Read the model definition and answer for the solid it produces. Units are mm, in the model's axes. Give positions to 0.01 mm unless a question says otherwise; leave off trailing zeros. Order: outer loops, then holes, each group sorted by start corner. A loop starts at its lowest first (then second) coordinate and runs counter-clockwise, first axis right, second up. Notation, with made-up numbers: (54, 26) -> (81, 26) arc R30 cw to (81, 62) -> close; hole circle Ø4 at (-6.5, 74.25). An arc over 180 degrees is marked (long way). One line per item, written item: value. Start each with the question number.
from build123d import *

# Parameters (mm, degrees)
SKETCH2_R           = 11
BOSS_EXTRUDE1_DEPTH = 7.5
SKETCH3_R           = 4.15
SKETCH3_R_2         = 1.25
CUT_EXTRUDE1_DEPTH  = 8.5


with BuildPart() as part:
    # Sketch2 → Boss-Extrude1 (new body)
    with BuildSketch(Plane.XY):
        Circle(SKETCH2_R)
    extrude(amount=BOSS_EXTRUDE1_DEPTH)

    # Sketch3 → Cut-Extrude1 (cut, through all)
    with BuildSketch(Plane(origin=(0, 0, 0), x_dir=(-1, 0, 0), z_dir=(0, 0, -1))):
        Circle(SKETCH3_R)
        with Locations((8, 0)):
            Circle(SKETCH3_R_2)
        with Locations((5.656854249, -5.656854249)):
            Circle(SKETCH3_R_2)
        with Locations((0, -8)):
            Circle(SKETCH3_R_2)
        with Locations((-5.656854249, -5.656854249)):
            Circle(SKETCH3_R_2)
        with Locations((-8, 0)):
            Circle(SKETCH3_R_2)
        with Locations((-5.656854249, 5.656854249)):
            Circle(SKETCH3_R_2)
        with Locations((0, 8)):
            Circle(SKETCH3_R_2)
        with Locations((5.656854249, 5.656854249)):
            Circle(SKETCH3_R_2)
    extrude(amount=-CUT_EXTRUDE1_DEPTH, mode=Mode.SUBTRACT)


solid = part.part
Item 1: Find section C-C on x = 3. Write down the section's boundary in (y, z).
Item 2: Find section D-D on y = -8.75. Write down the section's boundary in (x, z), then the cut area to 3 significant figures.
Item 3: Find the intervals of material crossed by line 1 (Y direction, x = 0, z = 1.75); line 2 (Y direction, x = 6, z = 5); line 3 (X direction, y = 5.5, z = 5.5), in increasing order. Write a range as from..to.
Item 4: Flat-ended cylindrical pins translate along their axes: pin 1 (2 mm diameter, centred on x = 0, y = -8, fed in from +Z); pin 2 (1 mm diameter, centred on y = -6, z = 3.5, fed in from +X); pin 3 (1 mm diameter, centred on y = 8, z = 4.5, fed in from +X); pin 4 (4 mm diameter, centred on y = 7, z = 2.5, fed in from -X). Find the tip coordinate at first contact, or state that the pin passes through.
Item 5: For a pull along Y with two mould halves and no side action, classify faces 1 (the flat face through (0, -5, 7.5)), 2 (the cylindrical face through (-2.38, -10.74, 3.7)), 3 (the cylindrical face through (-6.75, 0.05, 3.7)) as +Y half, -Y half, draft (parallel to the pull), parting line (faces both ways), or undercut.
Item 6: Find section A-A on x = 0. Write down the section's boundary in (y, z), then the cut area to 4 significant figures.
Checks:
1. outline: (-10.58, 0) -> (-2.87, 0) -> (-2.87, 7.5) -> (-10.58, 7.5) -> close; (2.87, 0) -> (10.58, 0) -> (10.58, 7.5) -> (2.87, 7.5) -> close
2. outline: (-6.67, 0) -> (-1, 0) -> (-1, 7.5) -> (-6.67, 7.5) -> close; (1, 0) -> (6.67, 0) -> (6.67, 7.5) -> (1, 7.5) -> close
2. area: 85.0 mm2
3. line 1: -11..-9.25, -6.75..-4.15, 4.15..6.75, 9.25..11
3. line 2: -9.22..-6.86, -4.45..4.45, 6.86..9.22
3. line 3: -9.53..-6.9, -4.42..4.42, 6.9..9.53
4. pin 1: through
4. pin 2: x = 9.53
4. pin 3: x = 8.05
4. pin 4: x = -9.8
5. face 1: draft
5. face 2: parting line
5. face 3: undercut
6. outline: (-11, 0) -> (-9.25, 0) -> (-9.25, 7.5) -> (-11, 7.5) -> close; (-6.75, 0) -> (-4.15, 0) -> (-4.15, 7.5) -> (-6.75, 7.5) -> close; (4.15, 0) -> (6.75, 0) -> (6.75, 7.5) -> (4.15, 7.5) -> close; (9.25, 0) -> (11, 0) -> (11, 7.5) -> (9.25, 7.5) -> close
6. area: 65.25 mm2
